from build123d import *

# Parameters (mm, degrees)
SKETCH1_W                = 17
SKETCH1_H                = 20
BOSS_EXTRUDE1_DEPTH      = 2
BOSS_EXTRUDE1_2_DEPTH    = 2
BOSS_EXTRUDE2_DEPTH      = 9
BOSS_EXTRUDE2_DEPTH_BACK = 9
SKETCH2_R                = 1.414213562


with BuildPart() as part:
    # Sketch1 → Boss-Extrude1 (new body)
    with BuildSketch(Plane(origin=(0, 0, 0), x_dir=(0, 1, 0), z_dir=(0, 0, 1))):
        with Locations((-9.5, 0)):
            Rectangle(SKETCH1_W, SKETCH1_H)
    extrude(amount=BOSS_EXTRUDE1_DEPTH)



with BuildPart() as body_2:
    # Sketch1 → Boss-Extrude1 2 (new body)
    with BuildSketch(Plane(origin=(0, 0, 0), x_dir=(0, 1, 0), z_dir=(0, 0, 1))):
        with Locations((9.5, 0)):
            Rectangle(SKETCH1_W, SKETCH1_H)
    extrude(amount=BOSS_EXTRUDE1_2_DEPTH)


with BuildPart() as part_1:
    add(part.part)

    add(body_2.part)  # Boss-Extrude2 merges body 2
    # Sketch2 → Boss-Extrude2 (add, two sides: drawn at the far end of the back side and taken through both)
    with BuildSketch(Plane.YZ.offset(-BOSS_EXTRUDE2_DEPTH_BACK)):
        with Locations((0, 1)):
            Circle(SKETCH2_R)
    extrude(amount=BOSS_EXTRUDE2_DEPTH + BOSS_EXTRUDE2_DEPTH_BACK)


solid = part_1.part
Design review of the part built by this model. Coordinates are the model's own, in mm. A direction names the side the tool comes from. Round coordinates to 2 decimals unless told otherwise and drop trailing zeros. Order: outer loops, then holes, each group sorted by start corner. A loop starts at its lowest first (then second) coordinate and runs counter-clockwise, first axis right, second up.
1) Machinability: for faces 4 (the flat face through (-9.5, 1, 1)), 5 (the flat face through (0, 9, 0)), 6 (the flat face through (0, 9, 2)), which of the approach directions +Z, -Z, +X, -X, +Y, -Y give a long, thin tool a straight path to every point of the face, cutting with its end or side? Answer none if there is none.
The answers:
face 4: +Z, -Z, -X
face 5: -Z, +X, -X, +Y
face 6: +Z, +X, -X, +Y
2) For L1, parallel to Z at x = 0.25, y = 3.5; L2, parallel to X at y = -0.5, z = 1.4; L3, parallel to Y at x = 6.25, z = 2.15, list the stretches that pass through material, from the lowest coordinate up.
The answers:
L1: z = 0 to 2
L2: x = -9 to 9
L3: y = -0.82 to 0.82
3) Consider section A-A (x = 4.75). State the section outline as (y, z) points.
The answers:
outline: (-18, 0) - (-1, 0) arc R1.41 ccw to (1, 0) - (18, 0) - (18, 2) - (1, 2) arc R1.41 ccw to (-1, 2) - (-18, 2) - close
4) Consider section C-C (y = 6.5). State the section outline as (x, z) points, plus the area to 3 significant figures.
The answers:
outline: (-10, 0) - (10, 0) - (10, 2) - (-10, 2) - close
area: 40.0 mm2
5) Draft analysis for pull direction Y (two halves, no side actions). For faces 1 (the flat face through (0, -10, 2)), 2 (the flat face through (9, 0, 1)), 3 (the flat face through (0, -18, 1)), state which applies: released by +Y, released by -Y, zero draft, split by the parting line, or undercut.
The answers:
face 1: zero draft
face 2: undercut
face 3: released by -Y
6) Consider section B-B (y = 0). State the section outline as (x, z) points.
The answers:
outline: (-9, -0.41) - (9, -0.41) - (9, 2.41) - (-9, 2.41) - close
7) Clearance check with flat-ended pins moving along their axes: pin 1 Ø4 at (x, y) = (7, 9.5) entering from -Z; pin 2 Ø10 at (x, y) = (-1, 9) entering from +Z. State where each tip first meets the part, or that it passes through.
The answers:
pin 1: stops at z = 0
pin 2: stops at z = 2
